Check sheet for the modelled part. Datum: model origin and axes. Units: mm. Round coordinates to 2 decimals unless told otherwise and drop trailing zeros. Loops run counter-clockwise (first coordinate to the right, second up) from the corner with the lowest first, then second, coordinate; pieces in that order, holes last. Notation, with made-up numbers: M 28,-14 L 78,-14 A21 cw 78,-8 Z; hole C -31.75,79 d4. An arc over 180 degrees is marked long. One line per question, with ' | ' between items. Start each with the question number.
(1) Section check C-C (x = 26.25). Count the separate pieces of the cut face and the enclosed holes in it, and give its area (3 significant figures).
(2) Go/stop test with a flat-tipped pin: P1, Ø1.6, axis at x = 27, z = -6.5, coming from the -Y side (3 decimals). Record where the tip stops, or that it passes through.
(3) Section check D-D (z = -39). Record the boundary of the cut face in (x, y) (3 decimals).
(4) Section check A-A (z = -6.35). Record the boundary of the cut face in (x, y) (3 decimals).
(5) Thickness scan on probe 1 along Y at (x, z) = (26.7, -6.35) (3 decimals); probe 2 along Z at (x, y) = (28.05, -11.5); probe 3 along Y at (x, z) = (26.1, -55.5). Record the ranges inside material, lowest first. Write a range as [from, to].
(6) Draft check along Z on faces 1 (the face through (26.97, -11.79, -5.17)), 2 (the face through (27.01, 3.89, -13.46)), 3 (the face through (27, 0, 0)), 4 (the face through (27, -15.875, -7)). Enter one of: +Z half, -Z half, draft (parallel to the pull), parting line (faces both ways), or undercut.
(7) Section check B-B (y = 2). Record the boundary of the cut face in (x, z) (3 decimals), and give its area (3 significant figures).
```python
from build123d import *

# Parameters (mm, degrees)
SKETCH3_W                = 114.3
SKETCH3_H                = 88.9
SKETCH3_W_2              = 95.25
SKETCH3_H_2              = 76.2
BOSS_EXTRUDE1_DEPTH      = 12.7
BOSS_EXTRUDE1_DEPTH_BACK = 12.7
SKETCH4_W                = 114.3
SKETCH4_H                = 88.9
BOSS_EXTRUDE2_DEPTH      = 3.175
SKETCH5_W                = 114.3
SKETCH5_H                = 88.9
BOSS_EXTRUDE3_DEPTH      = 3.175
SKETCH7_W                = 41.275
SKETCH7_H                = 25.4
BOSS_EXTRUDE4_DEPTH      = 6.35
SKETCH6_R                = 9.9695
CUT_EXTRUDE1_DEPTH       = 115.3
SKETCH13_W               = 26.035
SKETCH13_H               = 25.4
BOSS_EXTRUDE5_DEPTH      = 4.064
SKETCH19_R               = 0.9525
CUT_EXTRUDE4_DEPTH       = 25.4
SKETCH20_R               = 1.905
CUT_EXTRUDE7_DEPTH       = 3.175
SKETCH23_R               = 5.08
SKETCH23_R_2             = 1.905
SKETCH23_R_3             = 2.38125
CUT_EXTRUDE8_DEPTH       = 3.175
BOSS_EXTRUDE6_DEPTH      = 25.4
BOSS_EXTRUDE7_DEPTH      = 3.175
SKETCH27_R               = 4.7625
CUT_EXTRUDE9_DEPTH       = 32.75
CUT_EXTRUDE9_DEPTH_BACK  = 83.55
SKETCH28_R               = 2.5527
CUT_EXTRUDE10_DEPTH      = 32.75
FILLET1_R                = 9.525
FILLET2_R                = 1.27
CUT_EXTRUDE11_START      = -31.75
SKETCH29_W               = 6.35
SKETCH29_H               = 5.08
CUT_EXTRUDE11_DEPTH      = 38.1


with BuildPart() as part:
    # Sketch3 → Boss-Extrude1 (new body, two sides)
    with BuildSketch(Plane(origin=(0, 0, 0), x_dir=(1, 0, 0), z_dir=(0, 1, 0))) as boss_extrude1_sk:
        with Locations((0, -44.45)):
            Rectangle(SKETCH3_W, SKETCH3_H)
        with Locations((0, -44.45)):
            Rectangle(SKETCH3_W_2, SKETCH3_H_2, mode=Mode.SUBTRACT)
    extrude(amount=BOSS_EXTRUDE1_DEPTH)
    extrude(boss_extrude1_sk.sketch, amount=-BOSS_EXTRUDE1_DEPTH_BACK)

    # Sketch4 → Boss-Extrude2 (add)
    with BuildSketch(Plane.XZ.offset(12.7)):
        with Locations((0, 44.45)):
            Rectangle(SKETCH4_W, SKETCH4_H)
    extrude(amount=BOSS_EXTRUDE2_DEPTH)

    # Sketch7 → Boss-Extrude4 (add)
    with BuildSketch(Plane(origin=(0, -12.7, 0), x_dir=(1, 0, 0), z_dir=(0, 1, 0))):
        with Locations((-26.9875, -50.8)):
            Rectangle(SKETCH7_W, SKETCH7_H)
        with Locations((26.9875, -50.8)):
            Rectangle(SKETCH7_W, SKETCH7_H)
    extrude(amount=BOSS_EXTRUDE4_DEPTH)

    # Sketch6 → Cut-Extrude1 (cut, through all)
    with BuildSketch(Plane.ZY.offset(57.15)):
        with Locations((50.8, 0)):
            Circle(SKETCH6_R)
    extrude(amount=-CUT_EXTRUDE1_DEPTH, mode=Mode.SUBTRACT)

    # Sketch13 → Boss-Extrude5 (add)
    with BuildSketch(Plane(origin=(0, -12.7, 0), x_dir=(1, 0, 0), z_dir=(0, 1, 0))):
        with Locations((-19.3675, -50.8)):
            Rectangle(SKETCH13_W, SKETCH13_H)
        with Locations((19.3675, -50.8)):
            Rectangle(SKETCH13_W, SKETCH13_H)
    extrude(amount=BOSS_EXTRUDE5_DEPTH)

    # Sketch19 → Cut-Extrude4 (cut)
    with BuildSketch(Plane(origin=(0, 12.7, 0), x_dir=(1, 0, 0), z_dir=(0, 1, 0))):
        with Locations((-53.975, -3.175)):
            Circle(SKETCH19_R)
        with Locations((53.975, -3.175)):
            Circle(SKETCH19_R)
        with Locations((-53.975, -85.725)):
            Circle(SKETCH19_R)
        with Locations((53.975, -85.725)):
            Circle(SKETCH19_R)
    extrude(amount=-CUT_EXTRUDE4_DEPTH, mode=Mode.SUBTRACT)

    # Sketch25 → Boss-Extrude6 (add, symmetric)
    with BuildSketch(Plane(origin=(0, 0, 0), x_dir=(0, 0, -1), z_dir=(1, 0, 0))):
        Polygon((0, -15.875), (0, 15.875), (9.525, 15.875), (12.7, 3.175), (12.7, -15.875), align=None)
    extrude(amount=BOSS_EXTRUDE6_DEPTH, both=True)

    # Sketch27 → Cut-Extrude9 (cut, two sides)
    with BuildSketch(Plane(origin=(25.4, 0, 0), x_dir=(0, 0, -1), z_dir=(1, 0, 0))) as cut_extrude9_sk:
        with Locations((6.35, -9.525)):
            Circle(SKETCH27_R)
        with Locations((6.35, 3.175)):
            Circle(SKETCH27_R)
    extrude(amount=CUT_EXTRUDE9_DEPTH, mode=Mode.SUBTRACT)
    extrude(cut_extrude9_sk.sketch, amount=-CUT_EXTRUDE9_DEPTH_BACK, mode=Mode.SUBTRACT)

    # Sketch29 → Cut-Extrude11 (cut)
    with BuildSketch(Plane(origin=(0, 0, 38.1), x_dir=(-1, 0, 0), z_dir=(0, 0, -1)).offset(CUT_EXTRUDE11_START)):
        with Locations((-26.3525, -12.7)):
            Rectangle(SKETCH29_W, SKETCH29_H)
        with Locations((-12.3825, -12.7)):
            Rectangle(SKETCH29_W, SKETCH29_H)
    cut_extrude11 = extrude(amount=CUT_EXTRUDE11_DEPTH, mode=Mode.SUBTRACT)

    # Mirror2: Cut-Extrude11 across plane
    add(cut_extrude11.mirror(Plane(origin=(0, 0, 0), x_dir=(0, 0, 1), z_dir=(1, 0, 0))), mode=Mode.SUBTRACT)


with BuildPart() as body_2:
    # Sketch5 → Boss-Extrude3 (new body)
    with BuildSketch(Plane(origin=(0, 12.7, 0), x_dir=(1, 0, 0), z_dir=(0, 1, 0))):
        with Locations((0, -44.45)):
            Rectangle(SKETCH5_W, SKETCH5_H)
    extrude(amount=BOSS_EXTRUDE3_DEPTH)

    # Sketch20 → Cut-Extrude7 (cut)
    with BuildSketch(Plane(origin=(0, 15.875, 0), x_dir=(1, 0, 0), z_dir=(0, 1, 0))):
        with Locations((-53.975, -3.175)):
            Circle(SKETCH20_R)
        with Locations((-53.975, -85.725)):
            Circle(SKETCH20_R)
        with Locations((53.975, -85.725)):
            Circle(SKETCH20_R)
        with Locations((53.975, -3.175)):
            Circle(SKETCH20_R)
    extrude(amount=-CUT_EXTRUDE7_DEPTH, mode=Mode.SUBTRACT)

    # Sketch23 → Cut-Extrude8 (cut)
    with BuildSketch(Plane(origin=(0, 15.875, 0), x_dir=(1, 0, 0), z_dir=(0, 1, 0))):
        with Locations((36.232509154, -69.504266718)):
            Circle(SKETCH23_R)
        with Locations((44.45, -62.808533435)):
            Circle(SKETCH23_R_2)
        with Locations((28.015018307, -76.2)):
            Circle(SKETCH23_R_2)
        with Locations((2.615018307, -60.427283435)):
            Circle(SKETCH23_R_3)
    extrude(amount=-CUT_EXTRUDE8_DEPTH, mode=Mode.SUBTRACT)


with BuildPart() as body_3:
    # Sketch26 → Boss-Extrude7 (new body)
    with BuildSketch(Plane(origin=(25.4, 0, 0), x_dir=(0, 0, -1), z_dir=(1, 0, 0))):
        Polygon((0, 15.875), (9.525, 15.875), (12.7, 3.175), (50.8, -14.2875), (76.2, -20.6375), (44.45, -20.6375), (12.7, -15.875), (0, -15.875), align=None)
    extrude(amount=BOSS_EXTRUDE7_DEPTH)

    # Sketch28 → Cut-Extrude10 (cut, through all)
    with BuildSketch(Plane.ZY.offset(-25.4)):
        with Locations((-6.35, 3.175)):
            Circle(SKETCH28_R)
        with Locations((-6.35, -9.525)):
            Circle(SKETCH28_R)
    extrude(amount=-CUT_EXTRUDE10_DEPTH, mode=Mode.SUBTRACT)

    # Fillet1
    fillet1_edges = [body_3.edges().sort_by_distance(p)[0] for p in [
        (26.9875, 3.175, -12.7),
        (26.9875, -14.2875, -50.8),
        (26.9875, -20.6375, -44.45),
        (26.9875, -15.875, -12.7),
    ]]
    fillet(fillet1_edges, radius=FILLET1_R)

    # Fillet2
    fillet2_edges = [body_3.edges().sort_by_distance(p)[0] for p in [
        (26.9875, 15.875, 0),
        (26.9875, -15.875, 0),
    ]]
    fillet(fillet2_edges, radius=FILLET2_R)


with BuildPart() as body_4:
    # Mirror1: mirrored copy
    add(body_3.part.mirror(Plane(origin=(0, 0, 0), x_dir=(0, 0, 1), z_dir=(1, 0, 0))))


solid = body_3.part
```
The answers:
1) separate pieces: 1 | enclosed holes: 2 | area: 924 mm²
2) P1: y = -15.875
3) outline: M 25.4,-19.82 L 28.575,-19.82 L 28.575,-8.879 L 25.4,-8.879 Z
4) outline: M 25.4,-15.875 L 28.575,-15.875 L 28.575,-12.078 L 25.4,-12.078 Z; M 25.4,-6.972 L 28.575,-6.972 L 28.575,0.622 L 25.4,0.622 Z; M 25.4,5.728 L 28.575,5.728 L 28.575,15.875 L 25.4,15.875 Z
5) probe 1: [-15.875, -12.078], [-6.972, 0.622], [5.728, 15.875] | probe 2: [-44.72, -7.97], [-4.73, 0] | probe 3: [-20.64, -15.46]
6) face 1: undercut | face 2: -Z half | face 3: +Z half | face 4: draft
7) outline: M 25.4,-15.548 L 28.575,-15.548 L 28.575,-8.616 L 25.4,-8.616 Z; M 25.4,-4.084 L 28.575,-4.084 L 28.575,0 L 25.4,0 Z | area: 35.0 mm²
